Design review of the part built by this model. Coordinates are the model's own, in mm. Give positions to 0.01 mm unless a question says otherwise; leave off trailing zeros. Use one line per item in the form item = value. Start each with the question number.
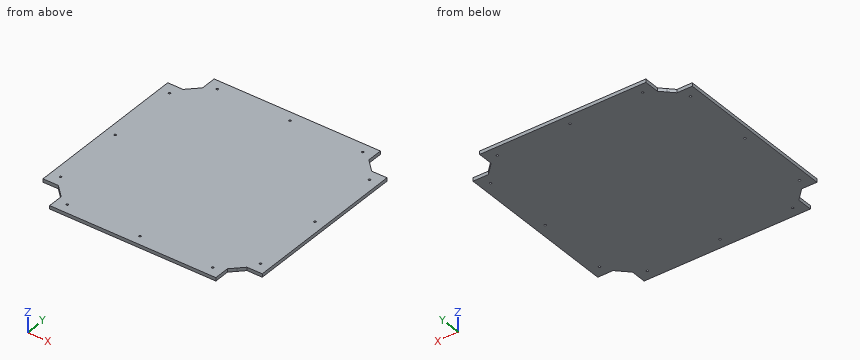
from build123d import *

# Parameters (mm, degrees)
F0_R     = 2.01
F1_DEPTH = 6.35


with BuildPart() as f1:
    # F0 (on Top) → F1 (new body)
    with BuildSketch(Plane.XY):
        Polygon((-158, 208.35), (-158, 194.175), (-158, 179.1715728753), (-168.5857864376, 168.5857864376), (-179.1715728753, 158), (-194.175, 158), (-208.35, 158), (-208.35, -158), (-194.175, -158), (-179.1715728753, -158), (-168.5857864376, -168.5857864376), (-158, -179.1715728753), (-158, -194.175), (-158, -208.35), (158, -208.35), (158, -194.175), (158, -179.1715728753), (168.5857864376, -168.5857864376), (179.1715728753, -158), (194.175, -158), (208.35, -158), (208.35, 158), (194.175, 158), (179.1715728753, 158), (168.5857864376, 168.5857864376), (158, 179.1715728753), (158, 194.175), (158, 208.35), align=None)
        with Locations((-138, -190)):
            Circle(F0_R, mode=Mode.SUBTRACT)
        with Locations((-190, -138)):
            Circle(F0_R, mode=Mode.SUBTRACT)
        with Locations((0, -190)):
            Circle(F0_R, mode=Mode.SUBTRACT)
        with Locations((138, -190)):
            Circle(F0_R, mode=Mode.SUBTRACT)
        with Locations((190, -138)):
            Circle(F0_R, mode=Mode.SUBTRACT)
        with Locations((-190, 0)):
            Circle(F0_R, mode=Mode.SUBTRACT)
        with Locations((-190, 138)):
            Circle(F0_R, mode=Mode.SUBTRACT)
        with Locations((-138, 190)):
            Circle(F0_R, mode=Mode.SUBTRACT)
        with Locations((190, 0)):
            Circle(F0_R, mode=Mode.SUBTRACT)
        with Locations((0, 190)):
            Circle(F0_R, mode=Mode.SUBTRACT)
        with Locations((190, 138)):
            Circle(F0_R, mode=Mode.SUBTRACT)
        with Locations((138, 190)):
            Circle(F0_R, mode=Mode.SUBTRACT)
    extrude(amount=F1_DEPTH)


solid = f1.part
Q1. Wall thickness on probe 1 along Y at (x, z) = (190, 5.25); probe 2 along Y at (x, z) = (0, 1.5): over which ranges is each line inside the solid? List them lowest first.
Q2. Take a section at A-A on z = 4.5. State how many separate pieces and enclosed holes the cut face has, plus the area to 3 significant figures.
Q3. Clearance check with flat-ended pins moving along their axes: pin 1 Ø1.9 at (x, z) = (-194, 2) entering from -Y; pin 2 Ø1.9 at (y, z) = (190.5, 2) entering from -X; pin 3 Ø1.5 at (x, z) = (163.5, 3) entering from -Y. State where each tip first meets the part, or that it passes through.
Response values:
q1.probe_1 = -158 to -140.01, -135.99 to -2.01, 2.01 to 135.99, 140.01 to 158
q1.probe_2 = -208.35 to -192.01, -187.99 to 187.99, 192.01 to 208.35
q2.separate_pieces = 1
q2.enclosed_holes = 12
q2.area = 164,000 mm^2
q3.pin_1 = -158
q3.pin_2 = -158
q3.pin_3 = -174.42
